For this review, take the finished solid that the model builds, in its own axes (mm). A direction names the side the tool comes from. Coordinates: 2 decimals unless noted, no trailing zeros. Loops run counter-clockwise (first coordinate to the right, second up) from the corner with the lowest first, then second, coordinate; pieces in that order, holes last. Notation, with made-up numbers: (-21, -27) -> (34, -27) arc R24 ccw to (34, 11) -> close; hole circle Ø7 at (47.25, 28.25). An arc over 180 degrees is marked (long way). One line per item, written item: value.
from build123d import *

# Parameters (mm, degrees)
F0_R     = 1.5875
F1_DEPTH = 3.175
F2_R     = 2.54


with BuildPart() as f1:
    # F0 (on Top) → F1 (new body)
    with BuildSketch(Plane.XY):
        Polygon((19.640194, 106.89594), (-38.779806, 48.47594), (-38.779806, 23.07594), (45.040194, 23.07594), (45.040194, 106.89594), align=None)
        with Locations((-30.340388, 35.77594)):
            Circle(F0_R, mode=Mode.SUBTRACT)
        with Locations((-6.210388, 35.77594)):
            Circle(F0_R, mode=Mode.SUBTRACT)
        with Locations((17.919612, 35.77594)):
            Circle(F0_R, mode=Mode.SUBTRACT)
        Polygon((17.919612, 48.47594), (-30.340388, 48.47594), (19.640194, 98.456522), align=None, mode=Mode.SUBTRACT)
    extrude(amount=F1_DEPTH)

    # F2
    f2_edges = [f1.edges().sort_by_distance(p)[0] for p in [
        (-30.340388, 48.47594, 1.5875),
        (17.919612, 48.47594, 1.5875),
        (19.640194, 98.456522, 1.5875),
    ]]
    fillet(f2_edges, radius=F2_R)


solid = f1.part
1. The part is to be moulded in two halves that separate along X. For faces 1 (the cylindrical face through (-26.57, 50.08, 1.61)), 2 (the flat face through (12, 47, 0)), 3 (the flat face through (45.04, 64, 2)), say which applies: pulls with the +X half, pulls with the -X half, needs draft (parallel to the pull), parting line crosses it, or undercut.
Return value:
face 1: undercut
face 2: needs draft
face 3: pulls with the +X half
2. To check wall thickness, follow probe 1 along X at (y, z) = (67, 2.2); probe 2 along Y at (x, z) = (-23.5, 1.95); probe 3 along Y at (x, z) = (2, 2.5). State the ranges of each line that lie inside material, in increasing order. Write a range as from..to.
Return value:
probe 1: x = -20.26..-11.82, 18.56..45.04
probe 2: y = 23.08..48.48, 55.32..63.76
probe 3: y = 23.08..48.48, 80.82..89.26
3. Take a section at A-A, the plane y = 76.5. Give the boundary of the cut face in (x, z) (3 decimals).
Return value:
outline: (-10.756, 0) -> (-2.316, 0) -> (-2.316, 3.175) -> (-10.756, 3.175) -> close; (18.884, 0) -> (45.04, 0) -> (45.04, 3.175) -> (18.884, 3.175) -> close
4. Take a section at C-C, the plane z = 2.35. Give the boundary of the cut face in (x, y) (1 decimal).
Return value:
outline: (-38.8, 23.1) -> (45, 23.1) -> (45, 106.9) -> (19.6, 106.9) -> (-38.8, 48.5) -> close; hole circle Ø3.2 at (-30.3, 35.8); hole (-26, 52.8) arc R2.5 ccw to (-24.2, 48.5) -> (15.5, 48.5) arc R2.5 ccw to (18, 50.9) -> (19.4, 92) arc R2.5 ccw to (15.1, 93.9) -> close; hole circle Ø3.2 at (-6.2, 35.8); hole circle Ø3.2 at (17.9, 35.8)
5. Insertion check: pin 1 Ø2.5 at (x, y) = (17.92, 35.78) entering from -Z; pin 2 Ø3.5 at (x, y) = (-6.21, 35.78) entering from -Z. Each pin has a flat end and moves straight along its axis. Give the tip position at first contact, or say it passes through.
Return value:
pin 1: passes through
pin 2: stops at z = 0
6. Take a section at B-B, the plane x = 4. Give the boundary of the cut face in (y, z) (3 decimals), and give its area (3 significant figures).
Return value:
outline: (23.076, 0) -> (48.476, 0) -> (48.476, 3.175) -> (23.076, 3.175) -> close; (82.816, 0) -> (91.256, 0) -> (91.256, 3.175) -> (82.816, 3.175) -> close
area: 107 mm2
7. For faces 4 (the flat face through (-9.161, 78.095, 1.565)), 5 (the cylindrical face through (17.931, 94.417, 1.61)), list the 3-axis set-ups (+Z, -Z, +X, -X, +Y, -Y) from which the entire face can be reached by the end or side of a thin tool; tool diameter is ignored.
Return value:
face 4: +Z, -Z, -X, +Y
face 5: +Z, -Z
